```python
from build123d import *

# Parameters (mm, degrees)
F0_W     = 160
F0_H     = 8
F1_DEPTH = 12
F2_DEPTH = 20
F3_W     = 8
F3_H     = 4
F4_DEPTH = 159.9984091469


with BuildPart() as f1:
    # F0 (on Front) → F1 (new body)
    with BuildSketch(Plane.XZ):
        Polygon((-65.9003738091, 63.3540591938), (-65.9003738091, -14.6459408062), (94.0996261909, -14.6459408062), (93.6557352543, 63.3540591938), align=None)
        Polygon((-85.9003738091, -14.6459408062), (-65.9003738091, -14.6459408062), (-65.9003738091, 63.3540591938), (93.6557352543, 63.3540591938), (94.0996261909, -14.6459408062), (114.0996261909, -14.6459408062), (114.0996261909, 75.3540591938), (94.0996261909, 75.3540591938), (94.0996261909, 67.3540591938), (-65.9003738091, 67.3540591938), (-65.9003738091, 75.3540591938), (-85.9003738091, 75.3540591938), align=None)
        with Locations((14.0996261909, 71.3540591938)):
            Rectangle(F0_W, F0_H)
    extrude(amount=F1_DEPTH)

    # F0 (on Front) → F2 (join)
    with BuildSketch(Plane.XZ):
        with Locations((14.0996261909, 71.3540591938)):
            Rectangle(F0_W, F0_H)
        Polygon((-65.9003738091, 63.3540591938), (-65.9003738091, -14.6459408062), (94.0996261909, -14.6459408062), (93.6557352543, 63.3540591938), align=None)
    extrude(amount=F2_DEPTH)

    # F3 (on face) → F4 (cut, through all)
    with BuildSketch(Plane(origin=(94.0132327131, 0, 0.5350207939), x_dir=(0, 1, 0), z_dir=(0.9999838072, 0, 0.0056908173))):
        with Locations((-16, -13.1812074268)):
            Rectangle(F3_W, F3_H)
    extrude(amount=-F4_DEPTH, mode=Mode.SUBTRACT)


solid = f1.part
```
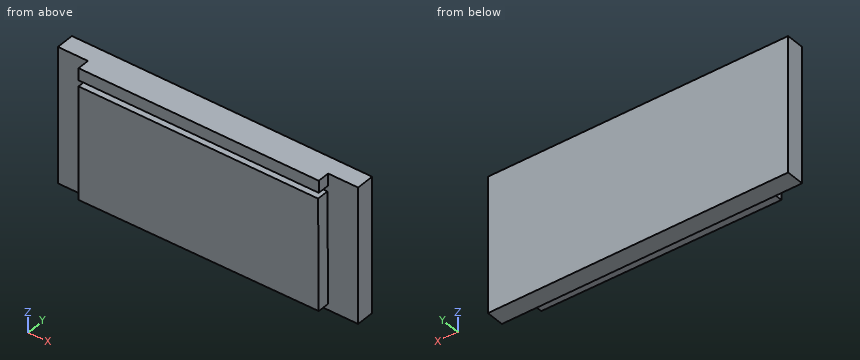
Check sheet for the modelled part. Datum: model origin and axes. Units: mm. Give positions to 0.01 mm unless a question says otherwise; leave off trailing zeros. Write each loop counter-clockwise with the first axis right and the second up, starting at its lowest first coordinate (ties: lowest second). Pieces come first, ordered by that corner, then holes. Notation, with made-up numbers: (88.5, -27.5) - (119.5, -27.5) arc R35 cw to (119.5, 8.5) - close; hole circle Ø10 at (-38.75, 0.25). An arc over 180 degrees is marked (long way). Answer as a JSON object with one key per item and string values. Group by question number.
1) Depth check by flat-ended pin: P1, Ø6.5, axis at y = -16, z = 70, coming from the -X side; P2, Ø6.5, axis at x = 16.5, y = -17.5, coming from the -Z side; P3, Ø4, axis at y = -15.5, z = 71, coming from the +X side. Enter the tip coordinate at first touch or a pass-through.
2) Sectioned sample at B-B (x = -26.5). Record the cut outline in (y, z), then the cut area to 3 significant figures.
3) Sectioned sample at A-A (y = -16). Record the cut outline in (x, z), then the cut area to 3 significant figures.
4) Sectioned sample at D-D (x = 76). Record the cut outline in (y, z).
5) Thickness scan on probe 1 along Y at (x, z) = (69, 64); probe 2 along Z at (x, y) = (-18.5, -17); probe 3 along X at (y, z) = (-16.25, 42). Record the ranges inside material, lowest first. Write a range as from..to.
6) Sectioned sample at C-C (z = 40.5). Record the cut outline in (x, y), then the cut area to 3 significant figures.
Geometry results:
{
 "1": {"P1": "stops at x = -65.9", "P2": "stops at z = -11.11", "P3": "stops at x = 94.1"},
 "2": {"outline": "(-20, -11.33) - (-12, -11.33) - (-12, -14.65) - (0, -14.65) - (0, 75.35) - (-20, 75.35) - (-20, 67.35) - (-12, 67.35) - (-12, 63.35) - (-20, 63.35) - close", "area": "1,740 mm^2"},
 "3": {"outline": "(-65.9, -11.56) - (94.08, -10.65) - (93.66, 63.35) - (-65.9, 63.35) - close; (-65.9, 67.35) - (94.1, 67.35) - (94.1, 75.35) - (-65.9, 75.35) - close", "area": "13,200 mm^2"},
 "4": {"outline": "(-20, -10.75) - (-12, -10.75) - (-12, -14.65) - (0, -14.65) - (0, 75.35) - (-20, 75.35) - (-20, 67.35) - (-12, 67.35) - (-12, 63.35) - (-20, 63.35) - close"},
 "5": {"probe 1": "y = -12..0", "probe 2": "z = -11.29..63.35, 67.35..75.35", "probe 3": "x = -65.9..93.78"},
 "6": {"outline": "(-85.9, -12) - (-65.9, -12) - (-65.9, -20) - (93.79, -20) - (93.79, -12) - (114.1, -12) - (114.1, 0) - (-85.9, 0) - close", "area": "3,680 mm^2"}
}
